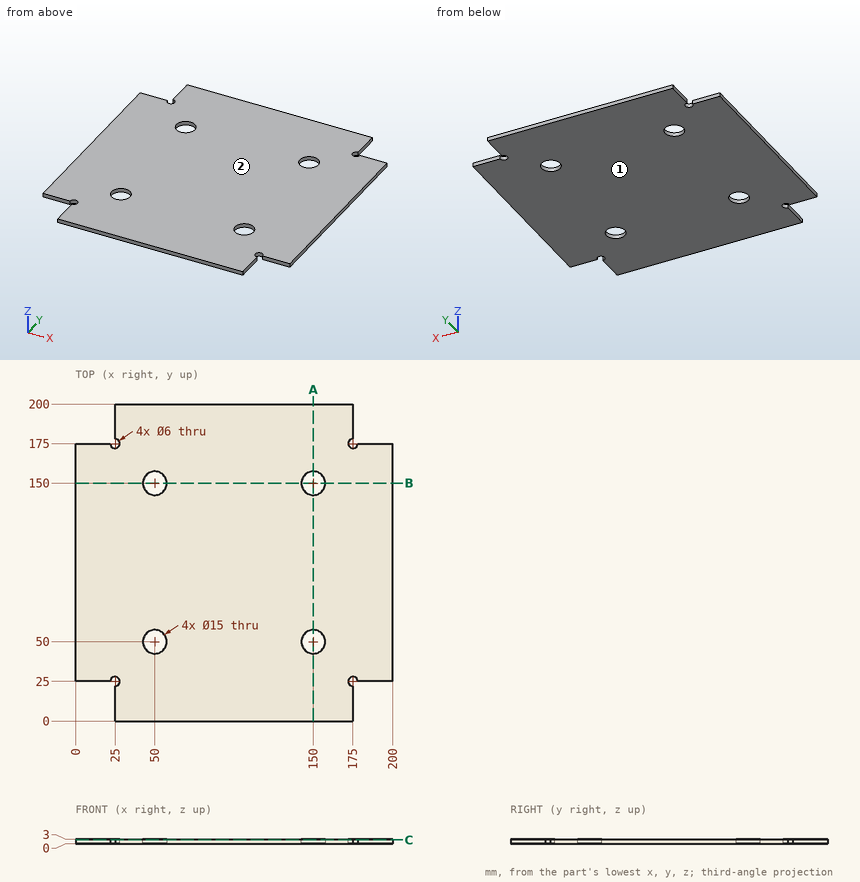
Answer from the drawing. Dimensions are ordinates in mm from the lowest x, y and z of the part. Round coordinates to 2 decimals unless told otherwise and drop trailing zeros. Order: outer loops, then holes, each group sorted by start corner. A loop starts at its lowest first (then second) coordinate and runs counter-clockwise, first axis right, second up.
1) Straight lines are drawn through the part: L1, parallel to X at y = 145, z = 0.9; L2, parallel to X at y = 181, z = 0.75. For each, find the intervals that lie inside material, in ascending order.
2) The part is cut by section C-C on z = 2.5. Write down the section's boundary in (x, y), plus the area to 3 significant figures.
3) The mould has two halves that part along Z. Classify the marked faces 1 and 2: released by +Z, released by -Z, zero draft, split by the parting line, or undercut.
4) Flat-ended cylindrical pins translate along their axes: pin 1 (1.5 mm diameter, centred on y = 12.5, z = 1, fed in from +X); pin 2 (0.9 mm diameter, centred on y = 187, z = 2, fed in from -X); pin 3 (0.9 mm diameter, centred on x = 188.5, z = 1, fed in from +Y). Find the tip coordinate at first contact, or state that the pin passes through.
5) The part is cut by section A-A on x = 150. Write down the section's boundary in (y, z), plus the area to 3 significant figures.
Resolved:
1. L1: x = 0 to 44.41, 55.59 to 144.41, 155.59 to 200
1. L2: x = 25 to 175
2. outline: (0, 25) - (22, 25) arc R3 cw (long way) to (25, 22) - (25, 0) - (175, 0) - (175, 22) arc R3 cw (long way) to (178, 25) - (200, 25) - (200, 175) - (178, 175) arc R3 cw (long way) to (175, 178) - (175, 200) - (25, 200) - (25, 178) arc R3 cw (long way) to (22, 175) - (0, 175) - close; hole circle Ø15 at (50, 50); hole circle Ø15 at (50, 150); hole circle Ø15 at (150, 50); hole circle Ø15 at (150, 150)
2. area: 36,700 mm2
3. face 1: released by -Z
3. face 2: released by +Z
4. pin 1: stops at x = 175
4. pin 2: stops at x = 25
4. pin 3: stops at y = 175
5. outline: (0, 0) - (42.5, 0) - (42.5, 3) - (0, 3) - close; (57.5, 0) - (142.5, 0) - (142.5, 3) - (57.5, 3) - close; (157.5, 0) - (200, 0) - (200, 3) - (157.5, 3) - close
5. area: 510 mm2
